Build history of the part. All positions in model axes, mm. A direction names the side the tool comes from. Give positions to 0.01 mm unless a question says otherwise; leave off trailing zeros. Order: outer loops, then holes, each group sorted by start corner. A loop starts at its lowest first (then second) coordinate and runs counter-clockwise, first axis right, second up. Notation, with made-up numbers: (-36.5, 75) -> (-17.5, 75) arc R37 ccw to (-17.5, 112) -> close; hole circle Ø11 at (54, 31.25). An arc over 180 degrees is marked (long way). Use a Markdown table: item, result. Add a question column.
```python
from build123d import *

# Parameters (mm, degrees)
ESQUISSE1_W        = 8
ESQUISSE1_H        = 6
BOSS_EXTRU_1_DEPTH = 6
ESQUISSE2_R        = 2
BOSS_EXTRU_2_DEPTH = 4


with BuildPart() as part:
    # Esquisse1 → Boss.-Extru.1 (new body)
    with BuildSketch(Plane.XY):
        Polygon((-8, 6), (0, 6), (0, 15), (-22, 15), (-22, 6), (-14, 6), align=None)
        with Locations((-4, 3)):
            Rectangle(ESQUISSE1_W, ESQUISSE1_H)
        with Locations((-18, 3)):
            Rectangle(ESQUISSE1_W, ESQUISSE1_H)
    extrude(amount=BOSS_EXTRU_1_DEPTH)

    # Esquisse2 → Boss.-Extru.2 (add)
    with BuildSketch(Plane.XY.offset(6)):
        with Locations((-12.403841621, 10)):
            Circle(ESQUISSE2_R)
    extrude(amount=BOSS_EXTRU_2_DEPTH)


solid = part.part
```
(1) Band-saw the part on D-D on x = -18.75. Give the cut face in (y, z), plus the area to 3 significant figures.
(2) Band-saw the part on A-A on y = 3. Give the cut face in (x, z), plus the area to 3 significant figures.
(3) Band-saw the part on B-B on z = 4.5. Give the cut face in (x, y).
(4) Pin check, flat tips, straight feed: pin 1 Ø3 at (x, z) = (-10.5, 1.5) entering from -Y; pin 2 Ø4.5 at (x, y) = (-6.5, 10.5) entering from +Z. Stop position of each tip, or through.
(5) Mould opens along X. For faces 1 (the face through (-14, 3, 3)), 2 (the face through (-11, 8, 0)), 3 (the face through (0, 7, 3)) say: released by +X, released by -X, zero draft, split by the parting line, or undercut.
(6) Tool access for faces 4 (the face through (-4, 0, 3)), 5 (the face through (-8, 3, 3)), 6 (the face through (-13.88, 11.35, 7.97)): list every direction of +Z, -Z, +X, -X, +Y, -Y with a clear straight run to the whole face (end or side of a thin tool).
(7) Wall check: probe 1 along X at (y, z) = (1.5, 1.5); probe 2 along Z at (x, y) = (-20, 10); probe 3 along Y at (x, z) = (-11.75, 0.5). Give the ranges that are in metal, low to high.
(8) Band-saw the part on C-C on y = 10. Give the cut face in (x, z).
Response:
| question | item | result |
|---|---|---|
| 1 | outline | (0, 0) -> (15, 0) -> (15, 6) -> (0, 6) -> close |
| 1 | area | 90.0 mm² |
| 2 | outline | (-22, 0) -> (-14, 0) -> (-14, 6) -> (-22, 6) -> close; (-8, 0) -> (0, 0) -> (0, 6) -> (-8, 6) -> close |
| 2 | area | 96.0 mm² |
| 3 | outline | (-22, 0) -> (-14, 0) -> (-14, 6) -> (-8, 6) -> (-8, 0) -> (0, 0) -> (0, 15) -> (-22, 15) -> close |
| 4 | pin 1 | stops at y = 6 |
| 4 | pin 2 | stops at z = 6 |
| 5 | face 1 | undercut |
| 5 | face 2 | zero draft |
| 5 | face 3 | released by +X |
| 6 | face 4 | +Z, -Z, +X, -X, -Y |
| 6 | face 5 | +Z, -Z, -Y |
| 6 | face 6 | +Z |
| 7 | probe 1 | x = -22 to -14, -8 to 0 |
| 7 | probe 2 | z = 0 to 6 |
| 7 | probe 3 | y = 6 to 15 |
| 8 | outline | (-22, 0) -> (0, 0) -> (0, 6) -> (-10.4, 6) -> (-10.4, 10) -> (-14.4, 10) -> (-14.4, 6) -> (-22, 6) -> close |
